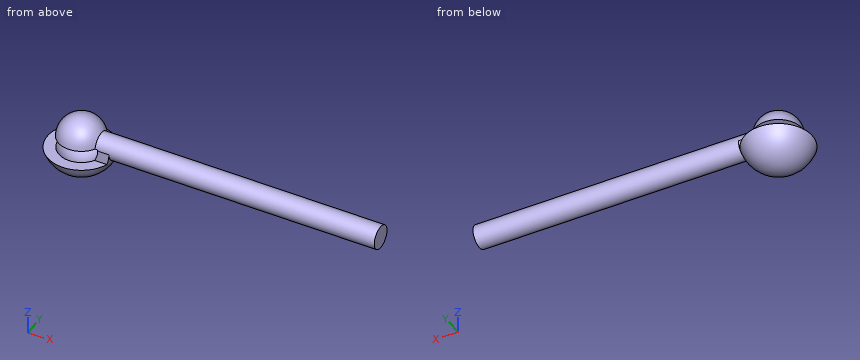
```python
from build123d import *

# Parameters (mm, degrees)
F2_R          = 10
F3_DEPTH      = 0.5
F3_DEPTH_BACK = 10.001
F6_R          = 5
F7_DEPTH      = 130
F11_DEPTH     = 5


with BuildPart() as f1:
    # F0 (on Front) → F1 (revolve)
    with BuildSketch(Plane.XZ):
        with BuildLine():
            Line((0, 10), (0, -10))
            ThreePointArc((0, -10), (10, 0), (0, 10))
        make_face()
    revolve(axis=Axis((0, 0, 0), (0, 0, -1)))

    # F2 (on Top) → F3 (cut, two sides)
    with BuildSketch(Plane.XY) as f3_sk:
        Circle(F2_R)
    extrude(amount=F3_DEPTH, mode=Mode.SUBTRACT)
    extrude(f3_sk.sketch, amount=-F3_DEPTH_BACK, mode=Mode.SUBTRACT)



with BuildPart() as f5:
    # F4 (on Front) → F5 (revolve)
    with BuildSketch(Plane.XZ):
        with BuildLine():
            ThreePointArc((11, 0), (7.7781745931, -7.7781745931), (0, -11))
            Line((0, -11), (0, -15.5))
            ThreePointArc((0, -15.5), (10.9601551084, -10.9601551084), (15.5, 0))
            Line((15.5, 0), (11, 0))
        make_face()
    revolve(axis=Axis((0, 0, -13.25), (0, 0, 1)))


with BuildPart() as f1_1:
    add(f1.part)

    add(f5.part)  # F7 merges F5
    # F6 (on Right) → F7 (join)
    with BuildSketch(Plane.YZ):
        Circle(F6_R)
    extrude(amount=F7_DEPTH)

    # F8 (on Front) → F9 (revolve, cut)
    with BuildSketch(Plane.XZ):
        with BuildLine():
            Line((0, 0.5), (0, -11))
            ThreePointArc((0, -11), (7.9529868603, -7.5993420768), (10.9886304879, 0.5))
            Line((10.9886304879, 0.5), (0, 0.5))
        make_face()
    revolve(axis=Axis((0, 0, -5.25), (0, 0, 1)), mode=Mode.SUBTRACT)

    # F10 (on Top) → F11 (cut)
    with BuildSketch(Plane.XY):
        with BuildLine():
            Line((0, 5), (14.6714007511, 5))
            ThreePointArc((14.6714007511, 5), (-15.5, 0), (14.6714007511, -5))
            Line((14.6714007511, -5), (0, -5))
            Line((0, -5), (0, 5))
        make_face()
    extrude(amount=-F11_DEPTH, mode=Mode.SUBTRACT)


solid = f1_1.part
```
Could you check a few things on this model? Use its own coordinates, in mm. Round coordinates to 2 decimals unless told otherwise and drop trailing zeros. Order: outer loops, then holes, each group sorted by start corner. A loop starts at its lowest first (then second) coordinate and runs counter-clockwise, first axis right, second up. Notation, with made-up numbers: M 67.5,80 L 101.5,80 A22 cw 101.5,98 Z; hole C -21.75,-33 d5. An arc over 180 degrees is marked long. One line per question, with ' | ' between items. Start each with the question number.
(1) Suppose I cut it at D-D on z = -7. List the corners of the cut face in (x, y) for me, then the cut area to 3 significant figures.
(2) Suppose I cut it at C-C on x = 56.5. List the corners of the cut face in (y, z) for me, then the cut area to 3 significant figures.
(3) For P1, Ø2, axis at x = 18.5, z = -3, coming from the -Y side; P2, Ø5, axis at y = 10, z = 0, coming from the +X side; P3, Ø6, axis at x = 3.5, y = -4.5, coming from the -Z side, each with a flat end and sliding along its axis, tell me the tip position at first contact or that it passes through.
(4) Suppose I cut it at A-A on y = 0. List the corners of the cut face in (x, z) for me.
(5) Please list where these lines run through material, in increasing order: line 1 along Z through (x, y) = (45, -0.5); line 2 along Y through (x, z) = (34.5, -0.25); line 3 along X through (y, z) = (-3.5, 4).
(6) Suppose I cut it at B-B on x = -4. List the corners of the cut face in (y, z) for me, then the cut area to 3 significant figures.
Geometry results:
1) outline: C 0,0 d27.66; hole C 0,0 d16.97 | area: 375 mm²
2) outline: C 0,0 d10 | area: 78.5 mm²
3) P1: y = -4.58 | P2: x = 6.54 | P3: z = -15.26
4) outline: M -14.67,-5 A15.5 ccw 14.67,-5 L 130,-5 L 130,5 L 8.66,5 A10 ccw -9.99,0.5 L 10.99,0.5 A11 cw -9.8,-5 Z
5) line 1: -4.97 to 4.97 | line 2: -4.99 to 4.99 | line 3: -8.47 to 8.47
6) outline: M -14.12,-5 A14.97 ccw 14.12,-5 L 8.94,-5 A10.25 cw -8.94,-5 Z; M -9.15,0.5 L 9.15,0.5 A9.17 ccw Z | area: 261 mm²
